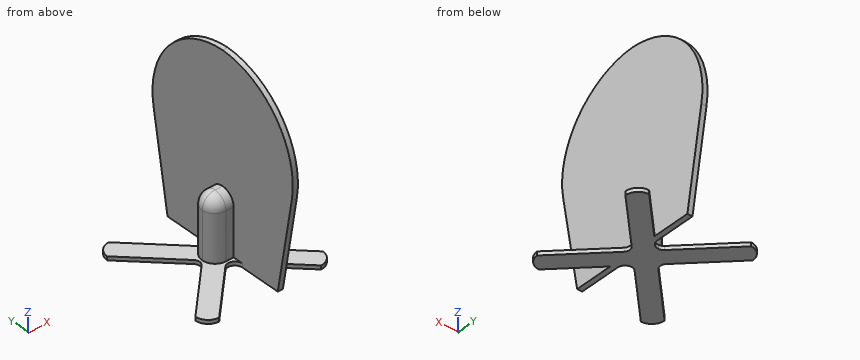
```python
from build123d import *

# Parameters (mm, degrees)
F1_DEPTH    = 3
F2_R        = 9.99999
F3_R        = 5
F4_DEPTH    = 50
F6_DEPTH    = 10
F7_DEPTH    = 6
F8_T1_DEPTH = 387.2306894548
F9_R        = 9.99999
F10_R       = 5.99999


# Not quite as in the source:
# - a fillet or chamfer that OpenCascade refuses, or shapes differently, is made with other operations: its cross-section is extruded or revolved along the edge and cut away or added
# - a fillet or chamfer is up to 0.001 mm smaller than in the source, because OpenCascade refuses the exact size


with BuildPart() as f1:
    # F0 (on Top) → F1 (new body)
    with BuildSketch(Plane.XY):
        with BuildLine():
            Line((0, 10), (10, 0))
            ThreePointArc((10, 0), (7.0710678119, 7.0710678119), (0, 10))
        make_face()
        with BuildLine():
            Line((50, -40), (10, 0))
            ThreePointArc((10, 0), (7.0710678119, -7.0710678119), (0, -10))
            Line((0, -10), (40, -50))
            Line((40, -50), (50, -50))
            Line((50, -50), (50, -40))
        make_face()
        Polygon((0, -10), (10, 0), (0, 10), (-10, 0), align=None)
        with BuildLine():
            ThreePointArc((0, 10), (7.0710678119, 7.0710678119), (10, 0))
            Line((10, 0), (50, 40))
            Line((50, 40), (50, 50))
            Line((50, 50), (40, 50))
            Line((40, 50), (0, 10))
        make_face()
        with BuildLine():
            ThreePointArc((0, -10), (7.0710678119, -7.0710678119), (10, 0))
            Line((10, 0), (0, -10))
        make_face()
        with BuildLine():
            Line((-10, 0), (0, 10))
            ThreePointArc((0, 10), (-7.0710678119, 7.0710678119), (-10, 0))
        make_face()
        with BuildLine():
            ThreePointArc((-10, 0), (-7.0710678119, 7.0710678119), (0, 10))
            Line((0, 10), (-40, 50))
            Line((-40, 50), (-50, 50))
            Line((-50, 50), (-50, 40))
            Line((-50, 40), (-10, 0))
        make_face()
        with BuildLine():
            Line((-40, -50), (0, -10))
            ThreePointArc((0, -10), (-7.0710678119, -7.0710678119), (-10, 0))
            Line((-10, 0), (-50, -40))
            Line((-50, -40), (-50, -50))
            Line((-50, -50), (-40, -50))
        make_face()
        with BuildLine():
            ThreePointArc((-10, 0), (-7.0710678119, -7.0710678119), (0, -10))
            Line((0, -10), (-10, 0))
        make_face()
    extrude(amount=F1_DEPTH)

    # F2 (radius 10 in the source; OpenCascade refuses exactly that, so slightly less here)
    f2_edges = [f1.edges().sort_by_distance(p)[0] for p in [
        (-50, 50, 1.5),
        (-50, -50, 1.5),
        (50, -50, 1.5),
        (50, 50, 1.5),
    ]]
    fillet(f2_edges, radius=F2_R)

    # F3
    f3_edges = [f1.edges().sort_by_distance(p)[0] for p in [
        (10, 0, 1.5),
        (0, 10, 1.5),
        (-10, 0, 1.5),
        (0, -10, 1.5),
    ]]
    fillet(f3_edges, radius=F3_R)

    # F0 (on Top) → F4 (join)
    with BuildSketch(Plane.XY):
        with BuildLine():
            Line((0, 10), (10, 0))
            ThreePointArc((10, 0), (7.0710678119, 7.0710678119), (0, 10))
        make_face()
        Polygon((0, -10), (10, 0), (0, 10), (-10, 0), align=None)
        with BuildLine():
            ThreePointArc((0, -10), (7.0710678119, -7.0710678119), (10, 0))
            Line((10, 0), (0, -10))
        make_face()
        with BuildLine():
            Line((-10, 0), (0, 10))
            ThreePointArc((0, 10), (-7.0710678119, 7.0710678119), (-10, 0))
        make_face()
        with BuildLine():
            ThreePointArc((-10, 0), (-7.0710678119, -7.0710678119), (0, -10))
            Line((0, -10), (-10, 0))
        make_face()
    extrude(amount=F4_DEPTH)

    # F5 (on Right) → F6 (join)
    with BuildSketch(Plane.YZ):
        with BuildLine():
            Line((-70.7106781187, 120.7106781187), (0, 150))
            ThreePointArc((0, 150), (-37.3285426078, 146.4855717522), (-73.3452003698, 136.0657990677))
            Line((-73.3452003698, 136.0657990677), (-70.7106781187, 120.7106781187))
        make_face()
        Polygon((-64.6446609407, 85.3553390593), (0, 150), (-70.7106781187, 120.7106781187), align=None)
        Polygon((-50, 0), (0, 0), (0, 150), (-64.6446609407, 85.3553390593), align=None)
        Polygon((0, 150), (0, 0), (50, 0), (64.6446609407, 85.3553390593), align=None)
        Polygon((70.7106781187, 120.7106781187), (0, 150), (64.6446609407, 85.3553390593), align=None)
        with BuildLine():
            ThreePointArc((73.3452003698, 136.0657990677), (37.3285426078, 146.4855717522), (0, 150))
            Line((0, 150), (70.7106781187, 120.7106781187))
            Line((70.7106781187, 120.7106781187), (73.3452003698, 136.0657990677))
        make_face()
    extrude(amount=F6_DEPTH)

    # F7 (cut): a face of the model
    f7_faces = [f1.faces().sort_by_distance(p)[0] for p in [
        (0, 0, 80.6875743248),
    ]]
    extrude(f7_faces, amount=-F7_DEPTH, mode=Mode.SUBTRACT)

    # F8: fillet of radius 65 on 2 edges, made by hand

    # F8_s2 → F8_t1 (cut)
    with BuildSketch(Plane.YZ.offset(-185.6153447274)):
        with BuildLine():
            ThreePointArc((-62.6966411117, 74.0014474486), (-48.1162932181, 127.140168964), (2.0255781715, 149.9897423196))
            ThreePointArc((2.0255781715, 149.9897423196), (-36.3330590034, 146.6720845048), (-73.3452003698, 136.0657990677))
            Line((-73.3452003698, 136.0657990677), (-62.6966411117, 74.0014474486))
        make_face()
        with BuildLine():
            ThreePointArc((62.6966411117, 74.0014474486), (48.1162932181, 127.140168964), (-2.0255781715, 149.9897423196))
            ThreePointArc((-2.0255781715, 149.9897423196), (36.3330590034, 146.6720845048), (73.3452003698, 136.0657990677))
            Line((73.3452003698, 136.0657990677), (62.6966411117, 74.0014474486))
        make_face()
    extrude(amount=F8_T1_DEPTH, mode=Mode.SUBTRACT)

    # F9 (radius 10 in the source; OpenCascade refuses exactly that, so slightly less here)
    f9_edges = [f1.edges().sort_by_distance(p)[0] for p in [
        (-10, 0, 50),
        (3, 10, 50),
        (3, -10, 50),
    ]]
    fillet(f9_edges, radius=F9_R)

    # F10 (radius 6 in the source; OpenCascade refuses exactly that, so slightly less here)
    f10_edges = [f1.edges().sort_by_distance(p)[0] for p in [
        (6, 12.071068, 1.5),
        (6, -12.071068, 1.5),
    ]]
    fillet(f10_edges, radius=F10_R)


solid = f1.part
```
Here's how the part is built. I have some questions about the finished solid (model axes, mm). Coordinates: 2 decimals unless noted, no trailing zeros. Order: outer loops, then holes, each group sorted by start corner. A loop starts at its lowest first (then second) coordinate and runs counter-clockwise, first axis right, second up. Notation, with made-up numbers: M 57.25,-9 L 63.25,-9 A24 cw 63.25,12 Z; hole C 87.5,50.5 d9. An arc over 180 degrees is marked long. Answer as a JSON object with one key per item and string values. Group by question number.
(1) Suppose I cut it at D-D, the plane y = 43.5. Please give me the cut outline in (x, z).
(2) Suppose I cut it at A-A, the plane x = -27.5. Please give me the cut outline in (y, z), then the cut area to 3 significant figures.
(3) I need wall thicknesses on probe 1 along Z at (x, y) = (20, 14); probe 2 along X at (y, z) = (-38.5, 7.5); probe 3 along Z at (x, y) = (9.5, -13.5). Which ranges of each line are inside material? Lowest first, please.
(4) Suppose I cut it at C-C, the plane z = 14.5. Please give me the cut outline in (x, y).
(5) Suppose I cut it at B-B, the plane y = -34.5. Please give me the cut outline in (x, z), then the cut area to 3 significant figures.
(6) For pin 1 (4 mm diameter, centred on x = 21.5, y = 12, fed in from +Z); pin 2 (1 mm diameter, centred on x = 23, y = 12, fed in from -Z); pin 3 (1.8 mm diameter, centred on x = 4, z = 21.5, fed in from -Y); pin 4 (6.5 mm diameter, centred on x = 3, z = 20.5, fed in from +Y), each with a flat end and sliding along its axis, tell me the tip position at first contact or that it passes through.
Values found:
{
 "1": {"outline": "M -49.37,0 L -33.5,0 L -33.5,3 L -49.37,3 Z; M 6,0 L 10,0 L 10,132.02 L 6,132.02 Z; M 33.5,0 L 49.37,0 L 49.37,3 L 33.5,3 Z"},
 "2": {"outline": "M -37.5,0 L -17.5,0 L -17.5,3 L -37.5,3 Z; M 17.5,0 L 37.5,0 L 37.5,3 L 17.5,3 Z", "area": "120 mm^2"},
 "3": {"probe 1": "z = 0 to 3", "probe 2": "x = 6 to 10", "probe 3": "z = 0 to 148.27"},
 "4": {"outline": "M 0,-10 L 6,-10 L 6,-52.49 L 10,-52.49 L 10,52.49 L 6,52.49 L 6,10 L 0,10 A10 ccw Z"},
 "5": {"outline": "M -44.5,0 L -24.5,0 L -24.5,3 L -44.5,3 Z; M 6,0 L 10,0 L 10,139.2 L 6,139.2 Z; M 24.5,0 L 44.5,0 L 44.5,3 L 24.5,3 Z", "area": "677 mm^2"},
 "6": {"pin 1": "stops at z = 3", "pin 2": "passes through", "pin 3": "stops at y = -10", "pin 4": "stops at y = 53.73"}
}
